from build123d import *

# Parameters (mm, degrees)
F0_R        = 2.2
F1_DEPTH    = 17.5
F3_DEPTH    = 17.5
F4_T        = 2
F4_T3_DEPTH = 21.5
F5_T1_DEPTH = 17.5
F5_T3_DEPTH = 17.5
F5_T5_DEPTH = 17.5
F5_T7_DEPTH = 42.5
F5_T9_DEPTH = 27.8553390593
F7_D        = 32
F7_DEPTH    = 4
F7_TIP      = 9.6137699044
F8_D        = 2.5
F8_DEPTH    = 4
F8_TIP      = 0.7510757738


# Not quite as in the source:
# - a fillet or chamfer that OpenCascade refuses, or shapes differently, is made with other operations: its cross-section is extruded or revolved along the edge and cut away or added
# - a shell that OpenCascade refuses in one call is made with other operations: the cavity is built on its own and cut out


with BuildPart() as f1:
    # F0 (on Front) → F1 (new body)
    with BuildSketch(Plane.XZ):
        with BuildLine():
            Line((25.5, -19), (25.5, 23))
            Line((25.5, 23), (-21.5, 23))
            ThreePointArc((-21.5, 23), (-25.5, 19), (-21.5, 15))
            Line((-21.5, 15), (17.5, 15))
            Line((17.5, 15), (17.5, -19))
            ThreePointArc((17.5, -19), (21.5, -23), (25.5, -19))
        make_face()
        with Locations((21.5, -19)):
            Circle(F0_R, mode=Mode.SUBTRACT)
        with Locations((-21.5, 19)):
            Circle(F0_R, mode=Mode.SUBTRACT)
    extrude(amount=F1_DEPTH)

    # F2 (on Front) → F3 (join, through all)
    with BuildSketch(Plane.XZ):
        Polygon((17.5, -18.7826429341), (17.5, 15), (-17.5, 15), (-26.2, 6.3), (-26.2, -25.75), (-5, -25.75), (-5, -22.75), align=None)
    extrude(amount=F3_DEPTH)

    # F4: shell of thickness 2, made by hand


with BuildPart() as f4_core1:
    # F4_t2: copy of F1
    add(f1.part)

    # the walls: a layer under each face that stays
    f4_faces = [f4_core1.faces().sort_by_distance(p)[0] for p in [
        (25.5, -8.75, 2),
        (21.5, -8.75, -23),
        (2, -8.75, 23),
        (-0.35, 0, -1.375),
        (-0.35, -17.5, -1.375),
        (17.5, -8.75, -18.891321467),
        (-25.5, -8.75, 19),
        (-19.5, -8.75, 15),
        (19.3, -8.75, -19),
        (-23.7, -8.75, 19),
        (6.25, -8.75, -20.766321467),
        (-21.85, -8.75, 10.65),
        (-26.2, -8.75, -9.725),
        (-5, -8.75, -24.25),
    ]]
    thicken(f4_faces, amount=-F4_T, mode=Mode.SUBTRACT)

    # F4_s4 → F4_t3 (cut)
    with BuildSketch(Plane.XZ.offset(-2)):
        Polygon((17.4834729636, -18.8023390891), (19.5, -18.7826429341), (19.5, -16.3991357489), (17.1527036447, -16.813027428), align=None)
        Polygon((-17.5141421356, 14.9941421356), (-17.5, 17), (-12.6715728753, 17), (-16.0857864376, 13.5857864376), align=None)
        Polygon((-4.9765270364, -22.7696961551), (-5.3472963553, -20.780384494), (-7, -21.0718007376), (-7, -22.75), align=None)
    extrude(amount=F4_T3_DEPTH, mode=Mode.SUBTRACT)


with BuildPart() as f1_1:
    add(f1.part)

    # what is left inside the walls is the cavity
    f4_cavity = [f4_core1.part.solids().sort_by_distance(p)[0] for p in [
        (-0.35, -15.48, -10.166667),
    ]]
    add(f4_cavity, mode=Mode.SUBTRACT)

    # F5: fillet of radius 5 on 5 edges, made by hand

    # F5_s2 → F5_t1 (join)
    with BuildSketch(Plane.XZ):
        with BuildLine():
            ThreePointArc((18.307091383, -21.4094261897), (16.1468840352, -19.7684999194), (13.4477147235, -19.4971701618))
            Line((13.4477147235, -19.4971701618), (13.3608906347, -19.0047662853))
            Line((13.3608906347, -19.0047662853), (17.4131759112, -18.2902390576))
            Line((17.4131759112, -18.2902390576), (18, -18.7826429341))
            ThreePointArc((18, -18.7826429341), (18, -19), (18.7062049602, -21.108247916))
            Line((18.7062049602, -21.108247916), (18.307091383, -21.4094261897))
        make_face()
    extrude(amount=F5_T1_DEPTH)

    # F5_s4 → F5_t3 (join)
    with BuildSketch(Plane.XZ):
        with BuildLine():
            ThreePointArc((-23.8469891482, 8.6530108518), (-22.3858577587, 12.3711260424), (-24.1144546907, 15.972686559))
            Line((-24.1144546907, 15.972686559), (-23.7876478544, 16.3511007391))
            ThreePointArc((-23.7876478544, 16.3511007391), (-21.5, 15.5), (-17.5, 15.5))
            Line((-17.5, 15.5), (-17.1464466094, 14.6464466094))
            Line((-17.1464466094, 14.6464466094), (-23.4934357576, 8.2994574612))
            Line((-23.4934357576, 8.2994574612), (-23.8469891482, 8.6530108518))
        make_face()
    extrude(amount=F5_T3_DEPTH)

    # F5_s6 → F5_t5 (join)
    with BuildSketch(Plane.XZ):
        with BuildLine():
            ThreePointArc((-1.0199301517, -22.0482063006), (-3.5569146257, -23.311037583), (-5, -25.75))
            Line((-5, -25.75), (-5, -22.75))
            Line((-5, -22.75), (-1.0199301517, -22.0482063006))
        make_face()
    extrude(amount=F5_T5_DEPTH)

    # F5_s8 → F5_t7 (cut)
    with BuildSketch(Plane.XZ.offset(-12.5)):
        with BuildLine():
            ThreePointArc((25.5, 18), (24.0355339059, 21.5355339059), (20.5, 23))
            Line((20.5, 23), (25.5, 23))
            Line((25.5, 23), (25.5, 18))
        make_face()
    extrude(amount=F5_T7_DEPTH, mode=Mode.SUBTRACT)

    # F5_s10 → F5_t9 (cut)
    with BuildSketch(Plane.XZ.offset(-5.1776695297)):
        with BuildLine():
            ThreePointArc((-26.2, 4.2289321881), (-25.8193976626, 6.14234935), (-24.7355339059, 7.7644660941))
            Line((-24.7355339059, 7.7644660941), (-26.2, 6.3))
            Line((-26.2, 6.3), (-26.2, 4.2289321881))
        make_face()
    extrude(amount=F5_T9_DEPTH, mode=Mode.SUBTRACT)

    # F7
    with Locations(Plane.XZ.offset(17.5)):
        with Locations((0, 0)):
            Hole(F7_D / 2, depth=F7_DEPTH)
            with Locations((0, 0, -(F7_DEPTH + F7_TIP / 2))):  # 118° drill point
                Cone(0, F7_D / 2, F7_TIP, mode=Mode.SUBTRACT)

    # F8
    with Locations(Plane.XZ.offset(17.5)):
        with Locations((-15.2900823734, 15.2900823734), (-16.7099176266, -16.7099176266), (15.2900823734, -15.2900823734), (16.7099176266, 16.7099176266)):
            Hole(F8_D / 2, depth=F8_DEPTH)
            with Locations((0, 0, -(F8_DEPTH + F8_TIP / 2))):  # 118° drill point
                Cone(0, F8_D / 2, F8_TIP, mode=Mode.SUBTRACT)


solid = f1_1.part
Input: part model. Units: mm. Frame: model coordinates. A direction names the side the tool comes from. Round coordinates to 2 decimals unless told otherwise and drop trailing zeros. Order: outer loops, then holes, each group sorted by start corner. A loop starts at its lowest first (then second) coordinate and runs counter-clockwise, first axis right, second up. Notation, with made-up numbers: (70, -38.5) - (84, -38.5) arc R31 cw to (84, -5.5) - close; hole circle Ø11 at (-13, 59.25). An arc over 180 degrees is marked (long way). Answer as a JSON object with one key per item and string values. Group by question number.
(1) Material intervals for probe 1 along Y at (x, z) = (-2, -16.5); probe 2 along X at (y, z) = (-3.75, -7); probe 3 along X at (y, z) = (-10, 20.5), sorted ascending. Write a range as from..to.
(2) Pin query (flat end, axial travel): P1, Ø1, axis at x = 15, y = -12.5, coming from the -Z side; P2, Ø4, axis at x = 21.5, z = -19, coming from the +Y side. Return the tip coordinate at first contact, or that it passes through.
(3) Cut plane B-B (x = 21.5). Return loops of the section in (y, z).
(4) Cut plane C-C (y = -1). Return loops of the section in (x, z), then the cut area to 3 significant figures.
(5) Cut plane A-A (z = 19). Return loops of the section in (x, y).
(6) Draft query along Z for faces 1 (the face through (12, -17.5, -12)), 2 (the face through (0, -9, 23)), 3 (the face through (-17.3, -8.7, 19)). Return one class per face: released by +Z, released by -Z, zero draft, split by the parting line, or undercut.
(7) Cut plane D-D (z = 0). Return loops of the section in (x, y).
(8) Reachability of faces 4 (the face through (-1, -2, -2)), 5 (the face through (15.555, -16.486, 16.231)), 6 (the face through (-7, -9, -23)), 7 (the face through (-16, -16, -25.75)) from +Z, -Z, +X, -X, +Y, -Y: full face, straight path, thin tool, end or side. Return the list, or none.
Here are the results:
{
 "1": {"probe 1": "y = -17.5..-15.5, -2..0", "probe 2": "x = -26.2..-24.2, 23.5..25.5", "probe 3": "x = -25.21..-23.11, -19.89..-17.58, 23.5..24.83"},
 "2": {"P1": "stops at z = -19.56", "P2": "passes through"},
 "3": {"outline": "(-17.5, -23) - (0, -23) - (0, -21.2) - (-17.5, -21.2) - close; (-17.5, -16.8) - (0, -16.8) - (0, 22.9) - (-17.5, 22.9) - close; hole (-15.5, -14.8) - (-2, -14.8) - (-2, 21) - (-15.5, 21) - close"},
 "4": {"outline": "(-26.2, -25.75) - (-5, -25.75) arc R5 cw to (-1.02, -22.05) - (13.45, -19.5) arc R5 cw to (18.31, -21.41) arc R4 ccw to (25.5, -19) - (25.5, 18) arc R5 ccw to (20.5, 23) - (-21.5, 23) arc R4 ccw to (-24.11, 15.97) arc R5 cw to (-23.85, 8.65) - (-24.74, 7.76) arc R5 ccw to (-26.2, 4.23) - close; hole circle Ø4.4 at (-21.5, 19); hole circle Ø4.4 at (21.5, -19)", "area": "2,310 mm^2"},
 "5": {"outline": "(-25.5, -17.5) - (-23.7, -17.5) - (-23.7, 0) - (-25.5, 0) - close; (-19.3, -17.5) - (25.4, -17.5) - (25.4, 0) - (-19.3, 0) - close; hole (-17.3, -15.5) - (23.5, -15.5) - (23.5, -2) - (-17.3, -2) - close"},
 "6": {"face 1": "zero draft", "face 2": "released by +Z", "face 3": "undercut"},
 "7": {"outline": "(-26.2, -17.5) - (-16, -17.5) - (-16, -15.5) - (-24.2, -15.5) - (-24.2, -2) - (23.5, -2) - (23.5, -15.5) - (16, -15.5) - (16, -17.5) - (25.5, -17.5) - (25.5, 0) - (-26.2, 0) - close"},
 "8": {"face 4": "none", "face 5": "-Y", "face 6": "-Z", "face 7": "-Z, +X, -X, +Y, -Y"}
}
